Could you check a few things on this model? Use its own coordinates, in mm. A direction names the side the tool comes from. Coordinates: 2 decimals unless noted, no trailing zeros. Loops run counter-clockwise (first coordinate to the right, second up) from the corner with the lowest first, then second, coordinate; pieces in that order, holes last. Notation, with made-up numbers: (-18.5, 45.5) - (27.5, 45.5) arc R23 ccw to (27.5, 76.5) - close; hole circle Ø4 at (51.25, 15.25). An arc over 180 degrees is marked (long way). Use CSV: the item, a comma, the result in double quotes.
from build123d import *

# Parameters (mm, degrees)
SKETCH2_W           = 25
SKETCH2_H           = 53
SKETCH2_R           = 2.75
BOSS_EXTRUDE1_DEPTH = 8
BOSS_EXTRUDE2_DEPTH = 15
SKETCH4_R           = 5.15
CUT_EXTRUDE1_DEPTH  = 4.5
CHAMFER1_SIZE       = 1


with BuildPart() as part:
    # Sketch2 → Boss-Extrude1 (new body)
    with BuildSketch(Plane.XY):
        with Locations((12.5, 26.5)):
            Rectangle(SKETCH2_W, SKETCH2_H)
        with Locations((9, 44.7)):
            Circle(SKETCH2_R, mode=Mode.SUBTRACT)
        with Locations((9, 7.7)):
            Circle(SKETCH2_R, mode=Mode.SUBTRACT)
    extrude(amount=BOSS_EXTRUDE1_DEPTH)

    # Sketch3 → Boss-Extrude2 (add)
    with BuildSketch(Plane.XZ):
        Polygon((25, 2.75), (26.732050808, 1.75), (26.732050808, 6.25), (25, 5.25), align=None)
    extrude(amount=-BOSS_EXTRUDE2_DEPTH)

    # Sketch4 → Cut-Extrude1 (cut)
    with BuildSketch(Plane.XY.offset(8)):
        with Locations((9, 44.7)):
            Circle(SKETCH4_R)
        with Locations((9, 7.7)):
            Circle(SKETCH4_R)
    extrude(amount=-CUT_EXTRUDE1_DEPTH, mode=Mode.SUBTRACT)

    # Chamfer1
    chamfer1_edges = [part.edges().sort_by_distance(p)[0] for p in [
        (3.85, 44.7, 8),
        (3.85, 7.7, 8),
    ]]
    chamfer(chamfer1_edges, length=CHAMFER1_SIZE)


solid = part.part
(1) Please list where these lines run through material, in increasing order: line 1 (Y direction, x = 9, z = 6.2); line 2 (Y direction, x = 9, z = 2); line 3 (X direction, y = 44.7, z = 2.7).
Computed:
line 1,"y = 0 to 2.55, 12.85 to 39.55, 49.85 to 53"
line 2,"y = 0 to 4.95, 10.45 to 41.95, 47.45 to 53"
line 3,"x = 0 to 6.25, 11.75 to 25"
(2) Suppose I cut it at B-B (x = 9). Write out the boundary of the cut face in (y, z), plus the area to 3 significant figures.
Computed:
outline,"(0, 0) - (4.95, 0) - (4.95, 3.5) - (2.55, 3.5) - (2.55, 7) - (1.55, 8) - (0, 8) - close; (10.45, 0) - (41.95, 0) - (41.95, 3.5) - (39.55, 3.5) - (39.55, 7) - (38.55, 8) - (13.85, 8) - (12.85, 7) - (12.85, 3.5) - (10.45, 3.5) - close; (47.45, 0) - (53, 0) - (53, 8) - (50.85, 8) - (49.85, 7) - (49.85, 3.5) - (47.45, 3.5) - close"
area,"291 mm²"
(3) Suppose I cut it at D-D (y = 44.7). Write out the boundary of the cut face in (x, z).
Computed:
outline,"(0, 0) - (6.25, 0) - (6.25, 3.5) - (3.85, 3.5) - (3.85, 7) - (2.85, 8) - (0, 8) - close; (11.75, 0) - (25, 0) - (25, 8) - (15.15, 8) - (14.15, 7) - (14.15, 3.5) - (11.75, 3.5) - close"
(4) Suppose I cut it at C-C (z = 4.25). Write out the boundary of the cut face in (x, y), plus the area to 3 significant figures.
Computed:
outline,"(0, 0) - (26.73, 0) - (26.73, 15) - (25, 15) - (25, 53) - (0, 53) - close; hole circle Ø10.3 at (9, 7.7); hole circle Ø10.3 at (9, 44.7)"
area,"1,180 mm²"
(5) Suppose I cut it at A-A (y = 7.7). Write out the boundary of the cut face in (x, z), plus the area to 3 significant figures.
Computed:
outline,"(0, 0) - (6.25, 0) - (6.25, 3.5) - (3.85, 3.5) - (3.85, 7) - (2.85, 8) - (0, 8) - close; (11.75, 0) - (25, 0) - (25, 2.75) - (26.73, 1.75) - (26.73, 6.25) - (25, 5.25) - (25, 8) - (15.15, 8) - (14.15, 7) - (14.15, 3.5) - (11.75, 3.5) - close"
area,"139 mm²"
(6) Thinking about a two-plate mould opening in X: for faces 4 (the face through (26.732, 7, 4)), 5 (the face through (12, 27, 8)), 6 (the face through (4.91, 4.57, 5.27)), 7 (the face through (11, 42, 3.5)), which applies, +X half, -X half, draft (parallel to the pull), parting line (faces both ways), or undercut?
Computed:
face 4,"+X half"
face 5,"draft"
face 6,"undercut"
face 7,"undercut"
(7) Will these pins go through, and if not, where does the flat tip stop? pin 1 (1.5 mm diameter, centred on x = 22.5, y = 43.5, fed in from -Z); pin 2 (8 mm diameter, centred on x = 10.5, y = 6.5, fed in from +Z); pin 3 (9 mm diameter, centred on x = 9, y = 7.7, fed in from +Z); pin 4 (0.9 mm diameter, centred on x = 26, z = 4.5, fed in from +Y).
Computed:
pin 1,"stops at z = 0"
pin 2,"stops at z = 7.77"
pin 3,"stops at z = 3.5"
pin 4,"stops at y = 15"
(8) Which directions (+Z, -Z, +X, -X, +Y, -Y) give clear straight access to the entire face, cutting with the end or side of a thin tool? Please do faces 1 (the face through (13, 0, 4)), 2 (the face through (26, 15, 4)), 3 (the face through (8.33, 49.806, 5.274)).
Computed:
face 1,"+Z, -Z, +X, -X, -Y"
face 2,"+Z, -Z, +X, +Y"
face 3,"+Z"
